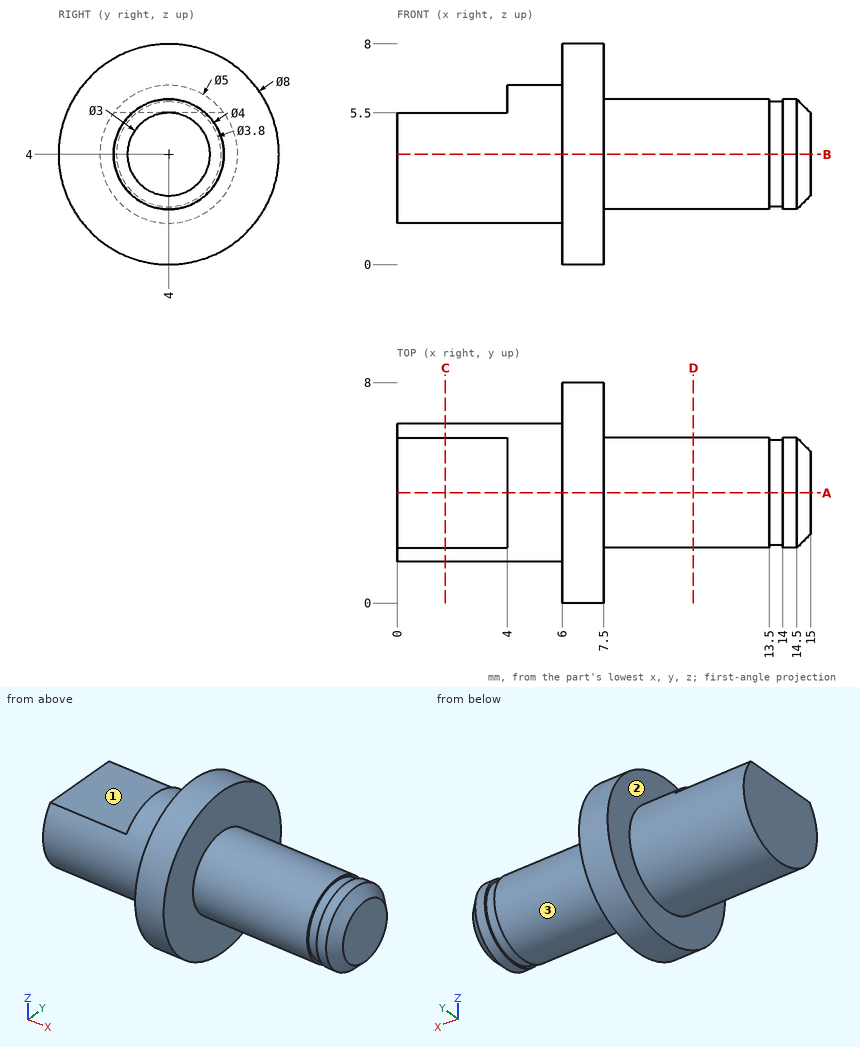
Print and shaded views of the part. All mm, measured from the part's lowest x, y and z. A direction names the side the tool comes from. Coordinates: 2 decimals unless noted, no trailing zeros. Loops run counter-clockwise (first coordinate to the right, second up) from the corner with the lowest first, then second, coordinate; pieces in that order, holes last. Notation, with made-up numbers: (61, -39.75) -> (75, -39.75) arc R25 ccw to (75, -20.75) -> close; hole circle Ø1 at (84.25, 42.5). An arc over 180 degrees is marked (long way). Use a Markdown table: item, result. Add a question column.
Item 1: Probe probe 1 along X at (y, z) = (3.25, 6.5); probe 2 along Z at (x, y) = (5.25, 2); probe 3 along X at (y, z) = (5, 2). List the from-to ranges inside material, lowest first.
Item 2: Which spindle directions (+Z, -Z, +X, -X, +Y, -Y) get a long thin tool onto all of the face, cutting with end or side? Do the marked faces 1, 2 and 3. Say none if no direction does.
Item 3: Band-saw the part on A-A on y = 4. Write the cut outline in (x, z).
Item 4: Flat gauge pins, fed straight in: P1, Ø4, axis at x = 13, y = 6, coming from the -Z side; P2, Ø4.5, axis at x = 2, y = 4, coming from the +Z side; P3, Ø1.1, axis at y = 4, z = 6, coming from the -X side. Where does each tip first touch, or does it go through?
Item 5: Band-saw the part on C-C on x = 1.75. Write the cut outline in (y, z).
Item 6: Band-saw the part on B-B on z = 4. Write the cut outline in (x, y), plus the area to 4 significant figures.
Item 7: Band-saw the part on D-D on x = 10.75. Write the cut outline in (y, z).
Geometry says:
| question | item | result |
|---|---|---|
| 1 | probe 1 | 6 to 7.5 |
| 1 | probe 2 | 2.5 to 5.5 |
| 1 | probe 3 | 0 to 7.5 |
| 2 | face 1 | +Z, -X, +Y, -Y |
| 2 | face 2 | -X |
| 2 | face 3 | +X |
| 3 | outline | (0, 1.5) -> (6, 1.5) -> (6, 0) -> (7.5, 0) -> (7.5, 2) -> (13.5, 2) -> (13.5, 2.1) -> (14, 2.1) -> (14, 2) -> (14.5, 2) -> (15, 2.5) -> (15, 5.5) -> (14.5, 6) -> (14, 6) -> (14, 5.9) -> (13.5, 5.9) -> (13.5, 6) -> (7.5, 6) -> (7.5, 8) -> (6, 8) -> (6, 6.5) -> (4, 6.5) -> (4, 5.5) -> (0, 5.5) -> close |
| 4 | P1 | z = 2 |
| 4 | P2 | z = 6.5 |
| 4 | P3 | x = 0 |
| 5 | outline | (2, 5.5) arc R2.5 ccw (long way) to (6, 5.5) -> close |
| 6 | outline | (0, 1.5) -> (6, 1.5) -> (6, 0) -> (7.5, 0) -> (7.5, 2) -> (13.5, 2) -> (13.5, 2.1) -> (14, 2.1) -> (14, 2) -> (14.5, 2) -> (15, 2.5) -> (15, 5.5) -> (14.5, 6) -> (14, 6) -> (14, 5.9) -> (13.5, 5.9) -> (13.5, 6) -> (7.5, 6) -> (7.5, 8) -> (6, 8) -> (6, 6.5) -> (0, 6.5) -> close |
| 6 | area | 71.65 mm² |
| 7 | outline | circle Ø4 at (4, 4) |
